```python
from build123d import *

# Parameters (mm, degrees)
SKETCH2_R           = 0.635
BOSS_EXTRUDE1_DEPTH = 2.54


with BuildPart() as part:
    # Sketch1 → Revolve1 (revolve)
    with BuildSketch(Plane.XY, mode=Mode.PRIVATE) as revolve1_sk:
        with BuildLine():
            Line((7.493, 0), (12.7, 0))
            Line((12.7, 0), (12.7, 12.7))
            Line((12.7, 12.7), (0, 12.7))
            Line((0, 12.7), (0, 7.493))
            ThreePointArc((0, 7.493), (5.298351111, 5.298351111), (7.493, 0))
        make_face()
    revolve(revolve1_sk.sketch.rotate(Axis((0, 12.7, 0), (0, -1, 0)), 180), axis=Axis((0, 12.7, 0), (0, -1, 0)))

    # Sketch2 → Boss-Extrude1 (add, symmetric)
    with BuildSketch(Plane.XY):
        with BuildLine():
            Line((-2.230711816, 20.264711816), (-6.35, 12.7))
            Line((-6.35, 12.7), (6.35, 12.7))
            Line((6.35, 12.7), (2.230711816, 20.264711816))
            ThreePointArc((2.230711816, 20.264711816), (0, 21.59), (-2.230711816, 20.264711816))
        make_face()
        with Locations((0, 19.05)):
            Circle(SKETCH2_R, mode=Mode.SUBTRACT)
    extrude(amount=BOSS_EXTRUDE1_DEPTH, both=True)


solid = part.part
```
Check sheet for the modelled part. Datum: model origin and axes. Units: mm. A direction names the side the tool comes from. Round coordinates to 2 decimals unless told otherwise and drop trailing zeros. Order: outer loops, then holes, each group sorted by start corner. A loop starts at its lowest first (then second) coordinate and runs counter-clockwise, first axis right, second up. Notation, with made-up numbers: M 36.25,56 L 86.25,56 A36 ccw 86.25,95 Z; hole C -35,-40 d5. An arc over 180 degrees is marked long. Answer in a Markdown table with one row per item.
(1) Section check A-A on x = 0. Record the boundary of the cut face in (y, z) (3 decimals), plus the area to 3 significant figures.
Findings:
| item | result |
|---|---|
| outline | M 0,-12.7 L 12.7,-12.7 L 12.7,-2.54 L 18.415,-2.54 L 18.415,2.54 L 12.7,2.54 L 12.7,12.7 L 0,12.7 L 0,7.493 A7.493 cw 0,-7.493 Z; M 19.685,-2.54 L 21.59,-2.54 L 21.59,2.54 L 19.685,2.54 Z |
| area | 273 mm^2 |
(2) Section check B-B on z = 0. Record the boundary of the cut face in (x, y) (3 decimals), plus the area to 3 significant figures.
Findings:
| item | result |
|---|---|
| outline | M -12.7,0 L -7.493,0 A7.493 cw 7.493,0 L 12.7,0 L 12.7,12.7 L 6.35,12.7 L 2.231,20.265 A2.54 ccw -2.231,20.265 L -6.35,12.7 L -12.7,12.7 Z; hole C 0,19.05 d1.27 |
| area | 302 mm^2 |
(3) Set-up check for faces 1 (the flat face through (0, 16, 2.54)), 2 (the cylindrical face through (-5.86, 6.439, 11.267)), 3 (the flat face through (0, 16, -2.54)): record each of +Z, -Z, +X, -X, +Y, -Y from which the full face is reachable in a straight line by a thin tool's end or side.
Findings:
| item | result |
|---|---|
| face 1 | +Z, +X, -X, +Y |
| face 2 | +Y, -Y |
| face 3 | -Z, +X, -X, +Y |
(4) Draft check along X on faces 4 (the flat face through (4.32, 16.43, 0.04)), 5 (the flat face through (-4.26, 16.54, 0.04)), 6 (the cylindrical face through (-0.14, 18.43, -0.04)). Enter one of: +X half, -X half, draft (parallel to the pull), parting line (faces both ways), or undercut.
Findings:
| item | result |
|---|---|
| face 4 | +X half |
| face 5 | -X half |
| face 6 | undercut |
(5) Section check C-C on y = 19.05. Record the boundary of the cut face in (x, z) (3 decimals).
Findings:
| item | result |
|---|---|
| outline | M -2.892,-2.54 L -0.635,-2.54 L -0.635,2.54 L -2.892,2.54 Z; M 0.635,-2.54 L 2.892,-2.54 L 2.892,2.54 L 0.635,2.54 Z |
(6) Material ranges on line 1 along Y through (x, z) = (8.25, 4.25); line 2 along Z through (x, y) = (-1.25, 19); line 3 along Z through (x, y) = (1.5, 9), recorded low to high. Write a range as from..to.
Findings:
| item | result |
|---|---|
| line 1 | y = 0..12.7 |
| line 2 | z = -2.54..2.54 |
| line 3 | z = -12.61..12.61 |
(7) Gauge pin test, flat ends, axial feed: pin 1 (10 mm diameter, centred on y = 9.5, z = -7.5, fed in from +X); pin 2 (8 mm diameter, centred on x = 4.5, y = 3.5, fed in from -Z); pin 3 (2 mm diameter, centred on x = 10, y = 7.5, fed in from -Z); pin 4 (1 mm diameter, centred on y = 15, z = -8, fed in from -X). Record the tip position at first contact, or that the pin passes through.
Findings:
| item | result |
|---|---|
| pin 1 | stops at x = 12.45 |
| pin 2 | stops at z = -12.69 |
| pin 3 | stops at z = -8.96 |
| pin 4 | passes through |
(8) Section check D-D on x = 3.75. Record the boundary of the cut face in (y, z).
Findings:
| item | result |
|---|---|
| outline | M 0,-12.13 L 12.7,-12.13 L 12.7,-2.54 L 17.47,-2.54 L 17.47,2.54 L 12.7,2.54 L 12.7,12.13 L 0,12.13 L 0,6.49 A6.49 cw 0,-6.49 Z |
